Source: CAD feature listing. Evaluate the final solid. Frame: model axes, mm. A direction names the side the tool comes from. Round coordinates to 2 decimals unless told otherwise and drop trailing zeros. Order: outer loops, then holes, each group sorted by start corner. A loop starts at its lowest first (then second) coordinate and runs counter-clockwise, first axis right, second up. Notation, with made-up numbers: (-36, 4.5) -> (-21, 4.5) arc R31 cw to (-21, 39.5) -> close; hole circle Ø7 at (4, -32.75). An arc over 180 degrees is marked (long way). One line per item, written item: value. Start each with the question number.
1) Section D-D (x = 35). Return the cut outline in (y, z).
2) Mould query, pull axis X, two halves, no side actions, for faces 3 (the face through (57.14, 1.97, 107.14)), 4 (the face through (0, 3, 42)), 5 (the face through (35, 60, 2)). Classes: pulls with the +X half, pulls with the -X half, needs draft (parallel to the pull), parting line crosses it, or undercut.
3) Section C-C (y = 30). Return the cut outline in (x, z).
4) Section A-A (z = 97.75). Return the cut outline in (x, y).
5) Section B-B (x = 50). Return the cut outline in (y, z), and give its area (3 significant figures).
6) Reachability of faces 1 (the face through (35, 34, 4)), 2 (the face through (70, 3, 42)) from +Z, -Z, +X, -X, +Y, -Y: full face, straight path, thin tool, end or side. Return the list, or none.
7) Pin query (flat end, axial travel): P1, Ø5.5, axis at x = 20, y = 30, coming from the -Z side; P2, Ø4, axis at x = 28.5, y = 9, coming from the -Z side; P3, Ø5, axis at x = 14.5, z = 85, coming from the +Y side; P4, Ø5, axis at x = 22.5, y = 35.5, coming from the +Z side. Return the tip coordinate at first contact, or that it passes through.
8) Ray query, L1, parallel to Z at x = 35, y = 1.5; L2, parallel to Y at x = 45.5, z = 22. Return the intervals inside material, ascending.
Autodesk Inventor part; units mm, degrees
ref_plane "YZ Plane" through (0, 0, 0) normal (1, 0, 0) x (0, 1, 0)
ref_plane "XZ Plane" through (0, 0, 0) normal (0, 1, 0) x (-1, 0, 0)
ref_plane "XY Plane" through (0, 0, 0) normal (0, 0, 1) x (1, 0, 0)
sketch "Sketch1" plane through (0, 0, 0) normal (0, 0, 1) x (1, 0, 0)
  line L0 (0, 0) -> (0, 60)
  line L1 (0, 60) -> (70, 60)
  line L2 (70, 60) -> (70, 0)
  line L3 (70, 0) -> (0, 0)
  dimension "d0" = 60
  dimension "d1" = 70
  dimension "d2" = 60
extrude "Extrusion1" add sketch "Sketch1" along normal blind 4
sketch "Sketch2" plane through (0, 0, 4) normal (0, 0, 1) x (1, 0, 0)
  line L0 (0, 0) -> (70, 0)
  line L1 (70, 0) -> (70, 60)
  line L2 (0, 0) -> (70, 0)
  line L3 (70, 0) -> (70, 4)
  line L4 (70, 4) -> (0, 4)
  line L5 (0, 4) -> (0, 0)
  dimension "d5" = 4
extrude "Extrusion2" add sketch "Sketch2" along normal blind 115
sketch "Sketch3" plane through (0, 0, 0) normal (0, 0, -1) x (-1, 0, 0)
  line L0 (-70, 60) -> (-70, 0)
  circle A0 centre (-50, 30) radius 3
  circle A1 centre (-20, 30) radius 3
  dimension "d15" = 6
  dimension "d16" = 6
extrude "Extrusion3" cut sketch "Sketch3" against normal blind 10
sketch "Sketch4" plane through (0, 0, 0) normal (0, -1, 0) x (1, 0, 0)
  line L0 (70, 0) -> (70, 119)
  line L1 (23, 0) -> (17, 0)
  line L2 (17, 0) -> (23, 0)
  circle A0 centre (50, 23) radius 3
  circle A1 centre (20, 23) radius 3
  dimension "d26" = 6
  dimension "d27" = 6
extrude "Extrusion4" cut sketch "Sketch4" against normal blind 10
sketch "Sketch5" plane through (0, 0, 0) normal (0, -1, 0) x (1, 0, 0)
  line L0 (70, 4) -> (70, 119)
  circle A0 centre (50, 23) radius 3
  circle A1 centre (35, 108.75) radius 5.25
  circle A2 centre (35, 86.75) radius 5.25
  circle A3 centre (35, 97.75) radius 4
  circle A4 centre (55.25, 86.75) radius 2
  circle A5 centre (55.25, 108.75) radius 2
  circle A6 centre (14.75, 86.75) radius 2
  circle A7 centre (14.75, 108.75) radius 2
  point P0 (0, 0)
  point P1 (20, 23)
  dimension "d36" = 8
  dimension "d41" = 4
  dimension "d42" = 4
  dimension "d43" = 4
  dimension "d44" = 4
extrude "Extrusion5" cut sketch "Sketch5" against normal blind 10 contours A1 | A2 | A3 | A4 | A5 | A6 | A7
sketch "Sketch6" plane through (70, 0, 0) normal (1, 0, 0) x (0, 0, -1)
  line L0 (0, 0) -> (-119, 0)
  line L1 (0, 4) -> (0, 4)
  line L2 (-4, 4) -> (-119, 4)
  line L3 (0, 60) -> (0, 0)
  line L4 (-4, 0) -> (-4, 0)
  arc A0 (-4, 0) -> (0, 4) centre (-4, 4) ccw
  line L5 (0, 4) -> (0, 0)
  line L6 (-4, 0) -> (0, 0)
  dimension "d47" = 4
  dimension "d48" = 4
  dimension "d49" = 4
extrude "Extrusion6" cut sketch "Sketch6" against normal blind 100
sketch "Sketch7" plane through (70, 60, 4) normal (1, 0, 0) x (0, 0, -1)
  line L0 (0, -56) -> (0, 0)
  line L1 (0, -52) -> (0, -52)
  line L2 (-4, -56) -> (-4, -56)
  arc A0 (-4, -56) -> (0, -52) centre (-4, -52) ccw
  line L3 (0, -52) -> (0, -56)
  line L4 (0, -56) -> (-115, -56)
  line L5 (-4, -56) -> (0, -56)
  point P0 (4, -60)
  dimension "d52" = 4
  dimension "d53" = 4
  dimension "d54" = 4
extrude "Extrusion7" add sketch "Sketch7" against normal blind 70
sketch "Sketch8" plane through (0, 0, 119) normal (0, -1, 0) x (1, 0, 0)
  circle A0 centre (35, -10.25) radius 5.25
  circle A1 centre (55.25, -32.25) radius 2
  circle A2 centre (55.25, -32.25) radius 2
  circle A3 centre (55.25, -10.25) radius 2
  circle A4 centre (55.25, -10.25) radius 2
  circle A5 centre (14.75, -10.25) radius 2
  circle A6 centre (14.75, -10.25) radius 2
  circle A7 centre (14.75, -32.25) radius 2
  circle A8 centre (14.75, -32.25) radius 2
  point P0 (0, -119)
extrude "Extrusion8" add sketch "Sketch8" against normal blind 4 contours A1 | A3 | A5 | A7
sketch "Sketch9" plane through (0, 0, 119) normal (0, -1, 0) x (1, 0, 0)
  circle A0 centre (35, -10.25) radius 5.25
  circle A1 centre (57.5, -10.25) radius 1.65
  circle A2 centre (12.5, -10.25) radius 1.65
  circle A3 centre (57.5, -32.25) radius 1.65
  circle A4 centre (12.5, -32.25) radius 1.65
  point P0 (0, -119)
  dimension "d62" = 3.3
  dimension "d63" = 3.3
  dimension "d66" = 3.3
  dimension "d67" = 3.3
extrude "Extrusion9" cut sketch "Sketch9" against normal blind 4 contours A1 | A2 | A3 | A4
Findings:
1. outline: (0, 4) arc R4 ccw to (4, 0) -> (60, 0) -> (60, 4) -> (8, 4) arc R4 cw to (4, 8) -> (4, 81.5) -> (0, 81.5) -> close; (0, 92) -> (4, 92) -> (4, 93.75) -> (0, 93.75) -> close; (0, 101.75) -> (4, 101.75) -> (4, 103.5) -> (0, 103.5) -> close; (0, 114) -> (4, 114) -> (4, 119) -> (0, 119) -> close
2. face 3: undercut
2. face 4: pulls with the -X half
2. face 5: needs draft
3. outline: (0, 0) -> (17, 0) -> (17, 4) -> (0, 4) -> close; (23, 0) -> (47, 0) -> (47, 4) -> (23, 4) -> close; (53, 0) -> (70, 0) -> (70, 4) -> (53, 4) -> close
4. outline: (0, 0) -> (31, 0) -> (31, 4) -> (0, 4) -> close; (39, 0) -> (70, 0) -> (70, 4) -> (39, 4) -> close
5. outline: (0, 4) arc R4 ccw to (4, 0) -> (27, 0) -> (27, 4) -> (8, 4) arc R4 cw to (4, 8) -> (4, 20) -> (0, 20) -> close; (0, 26) -> (4, 26) -> (4, 119) -> (0, 119) -> close; (33, 0) -> (60, 0) -> (60, 4) -> (33, 4) -> close
5. area: 652 mm2
6. face 1: +Z, +X, -X, +Y
6. face 2: +Z, -Z, +X, +Y, -Y
7. P1: through
7. P2: z = 0
7. P3: y = 4
7. P4: z = 4
8. L1: 0.88 to 81.5, 92 to 93.75, 101.75 to 103.5, 114 to 119
8. L2: 0 to 4
